For this review, take the finished solid that the model builds, in its own axes (mm). A direction names the side the tool comes from. Round coordinates to 2 decimals unless told otherwise and drop trailing zeros. Loops run counter-clockwise (first coordinate to the right, second up) from the corner with the lowest first, then second, coordinate; pieces in that order, holes last. Notation, with made-up numbers: (67.25, 35.5) -> (86.25, 35.5) arc R23 ccw to (86.25, 69.5) -> close; hole circle Ø2 at (69.25, 33.5). An arc over 180 degrees is marked (long way). Write each question's results on one line, items separated by ' | '.
```python
from build123d import *

# Parameters (mm, degrees)
SKETCH_1_R          = 20
SKETCH_1_R_2        = 7.5
SKETCH_1_R_3        = 1
EXTRUDE_1_DEPTH     = 2
SKETCH_2_R          = 12.5
SKETCH_2_R_2        = 7.5
EXTRUDE_2_DEPTH     = 5
SKETCH_3_R          = 13.5
SKETCH_3_R_2        = 12.5
EXTRUDE_3_DEPTH     = 0.9
SKETCH_4_W          = 9.188934261
SKETCH_4_H          = 4
CUT_EXTRUDE_1_DEPTH = 10
FILLET_1_R          = 1
HOLE_WIZARD_M3_1_D  = 2.5


with BuildPart() as part:
    # 草图1 → 凸台-拉伸1 (new body)
    with BuildSketch(Plane(origin=(0, 0, 0), x_dir=(1, 0, 0), z_dir=(0, 1, 0))):
        with Locations(Location((0, 0, 0), (0, 0, 270))):
            Circle(SKETCH_1_R)
        with Locations(Location((0, 0, 0), (0, 0, 270))):
            Circle(SKETCH_1_R_2, mode=Mode.SUBTRACT)
        with Locations(Location((0, 16.5, 0), (0, 0, 270))):
            Circle(SKETCH_1_R_3, mode=Mode.SUBTRACT)
        with Locations(Location((14.289419162, 8.25, 0), (0, 0, 270))):
            Circle(SKETCH_1_R_3, mode=Mode.SUBTRACT)
        with Locations(Location((14.289419162, -8.25, 0), (0, 0, 270))):
            Circle(SKETCH_1_R_3, mode=Mode.SUBTRACT)
        with Locations(Location((0, -16.5, 0), (0, 0, 270))):
            Circle(SKETCH_1_R_3, mode=Mode.SUBTRACT)
        with Locations(Location((-14.289419162, -8.25, 0), (0, 0, 270))):
            Circle(SKETCH_1_R_3, mode=Mode.SUBTRACT)
        with Locations(Location((-14.289419162, 8.25, 0), (0, 0, 270))):
            Circle(SKETCH_1_R_3, mode=Mode.SUBTRACT)
    extrude(amount=EXTRUDE_1_DEPTH)

    # 草图2 → 凸台-拉伸2 (add)
    with BuildSketch(Plane(origin=(0, 2, 0), x_dir=(1, 0, 0), z_dir=(0, 1, 0))):
        with Locations(Location((0, 0, 0), (0, 0, 270))):
            Circle(SKETCH_2_R)
        with Locations(Location((0, 0, 0), (0, 0, 270))):
            Circle(SKETCH_2_R_2, mode=Mode.SUBTRACT)
    extrude(amount=EXTRUDE_2_DEPTH)

    # 草图3 → 凸台-拉伸3 (add)
    with BuildSketch(Plane(origin=(0, 2, 0), x_dir=(1, 0, 0), z_dir=(0, 1, 0))):
        with Locations(Location((0, 0, 0), (0, 0, 270))):
            Circle(SKETCH_3_R)
        with Locations(Location((0, 0, 0), (0, 0, 270))):
            Circle(SKETCH_3_R_2, mode=Mode.SUBTRACT)
    extrude(amount=EXTRUDE_3_DEPTH)

    # 草图4 → 切除-拉伸1 (cut)
    with BuildSketch(Plane.XZ):
        with Locations((-18.59446713, 0)):
            Rectangle(SKETCH_4_W, SKETCH_4_H)
    extrude(amount=-CUT_EXTRUDE_1_DEPTH, mode=Mode.SUBTRACT)

    # 圆角1
    fillet_1_edges = [part.edges().sort_by_distance(p)[0] for p in [
        (-19.899748742, 1, -2),
        (-19.899748742, 1, 2),
        (-14, 1, 2),
        (-14, 1, -2),
    ]]
    fillet(fillet_1_edges, radius=FILLET_1_R)

    # M3 螺纹孔1 (through all)
    with Locations(Plane.XZ):
        with Locations((-14.289419162, 8.25), (0, 16.5), (14.289419162, 8.25), (14.289419162, -8.25), (0, -16.5), (-14.289419162, -8.25)):
            Hole(HOLE_WIZARD_M3_1_D / 2)


solid = part.part
```
1. Draft analysis for pull direction X (two halves, no side actions). For faces 4 (the face through (-17, 1, 2)), 5 (the face through (-13.18, 2.44, -2.93)), 6 (the face through (0.16, 1.01, -15.26)), state which applies: released by +X, released by -X, zero draft, split by the parting line, or undercut.
Values found:
face 4: zero draft | face 5: split by the parting line | face 6: undercut
2. To check wall thickness, follow probe 1 along Z at (x, y) = (-10, 6); probe 2 along Y at (x, z) = (12.5, -2); probe 3 along Z at (x, y) = (0.5, 4.25). State the ranges of each line that lie inside material, in increasing order.
Values found:
probe 1: z = -7.5 to 7.5 | probe 2: y = 0 to 2.9 | probe 3: z = -12.49 to -7.48, 7.48 to 12.49
3. Consider section D-D (x = -6). State the section outline as (y, z) points.
Values found:
outline: (0, -19.08) -> (2, -19.08) -> (2, -12.09) -> (2.9, -12.09) -> (2.9, -10.97) -> (7, -10.97) -> (7, -4.5) -> (0, -4.5) -> close; (0, 4.5) -> (7, 4.5) -> (7, 10.97) -> (2.9, 10.97) -> (2.9, 12.09) -> (2, 12.09) -> (2, 19.08) -> (0, 19.08) -> close
4. Tool access review of faces 1 (the face through (-9, 2.9, 9)), 2 (the face through (-14.285, 1.014, -1.699)), 3 (the face through (14.56, 1.01, -9.47)): name each direction out of +Z, -Z, +X, -X, +Y, -Y from which nothing blocks a thin tool from reaching the whole face with its end or side.
Values found:
face 1: +Y | face 2: -X, +Y, -Y | face 3: +Y, -Y
5. For pin 1 (1.5 mm diameter, centred on x = 1.5, y = 4, fed in from +Z); pin 2 (1.5 mm diameter, centred on x = 4, y = 1.5, fed in from -Z); pin 3 (0.6 mm diameter, centred on x = -17.5, y = 1.5, fed in from +Z), all flat-tipped, find the tip position at first contact; note any pin that passes through.
Values found:
pin 1: stops at z = 12.48 | pin 2: stops at z = -19.73 | pin 3: stops at z = 10.21
6. Consider section B-B (z = 17). State the section outline as (x, y) points, plus the area to 3 significant figures.
Values found:
outline: (-10.54, 0) -> (-1.15, 0) -> (-1.15, 2) -> (-10.54, 2) -> close; (1.15, 0) -> (10.54, 0) -> (10.54, 2) -> (1.15, 2) -> close | area: 37.6 mm2
7. Consider section A-A (x = 0). State the section outline as (y, z) points, plus the area to 3 significant figures.
Values found:
outline: (0, -20) -> (2, -20) -> (2, -17.75) -> (0, -17.75) -> close; (0, -15.25) -> (2, -15.25) -> (2, -13.5) -> (2.9, -13.5) -> (2.9, -12.5) -> (7, -12.5) -> (7, -7.5) -> (0, -7.5) -> close; (0, 7.5) -> (7, 7.5) -> (7, 12.5) -> (2.9, 12.5) -> (2.9, 13.5) -> (2, 13.5) -> (2, 15.25) -> (0, 15.25) -> close; (0, 17.75) -> (2, 17.75) -> (2, 20) -> (0, 20) -> close | area: 91.8 mm2
8. Consider section C-C (y = 1.5). State the section outline as (x, z) points.
Values found:
outline: (-19.75, -3.16) arc R20 ccw (long way) to (-19.75, 3.16) arc R1 ccw to (-18.76, 2) -> (-15, 2) arc R1 cw to (-14, 1) -> (-14, -1) arc R1 cw to (-15, -2) -> (-18.76, -2) arc R1 ccw to start; hole circle Ø2.5 at (-14.29, -8.25); hole circle Ø2.5 at (-14.29, 8.25); hole circle Ø15 at (0, 0); hole circle Ø2.5 at (0, -16.5); hole circle Ø2.5 at (0, 16.5); hole circle Ø2.5 at (14.29, -8.25); hole circle Ø2.5 at (14.29, 8.25)
